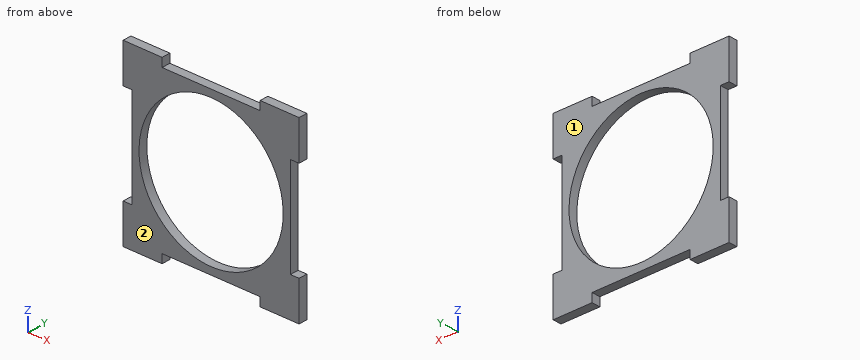
from build123d import *

# Parameters (mm, degrees)
CROQUIS1_R              = 25
SALIENTE_EXTRUIR1_DEPTH = 3


with BuildPart() as part:
    # Croquis1 → Saliente-Extruir1 (new body)
    with BuildSketch(Plane(origin=(0, 0, 0), x_dir=(1, 0, 0), z_dir=(0, 1, 0))):
        Polygon((-27.5, 0), (-27.5, 17), (-30.5, 17), (-30.5, 23.75), (-30.5, 30.5), (-23.75, 30.5), (-17, 30.5), (-17, 27.5), (0, 27.5), (17, 27.5), (17, 30.5), (23.75, 30.5), (30.5, 30.5), (30.5, 23.75), (30.5, 17), (27.5, 17), (27.5, 0), (27.5, -17), (30.5, -17), (30.5, -30.5), (23.75, -30.5), (17, -30.5), (17, -27.5), (0, -27.5), (-17, -27.5), (-17, -30.5), (-23.75, -30.5), (-30.5, -30.5), (-30.5, -23.75), (-30.5, -17), (-27.5, -17), align=None)
        with Locations(Location((0, 0, 0), (0, 0, 270))):
            Circle(CROQUIS1_R, mode=Mode.SUBTRACT)
    extrude(amount=SALIENTE_EXTRUIR1_DEPTH)


solid = part.part
Verification items for the finished model (mm, model axes). Face numbers are marked on the shaded views. Give positions to 0.01 mm unless a question says otherwise; leave off trailing zeros. Loops run counter-clockwise (first coordinate to the right, second up) from the corner with the lowest first, then second, coordinate; pieces in that order, holes last.
1) Thickness scan on line 1 along X through (y, z) = (0.6, 0); line 2 along Z through (x, y) = (0.5, 0.9) (3 decimals); line 3 along Z through (x, y) = (14.5, 0.8). Record the ranges inside material, lowest first.
2) Sectioned sample at C-C, the plane x = 23.5. Enter the section's corners in (y, z), then the cut area to 3 significant figures.
3) Depth check by flat-ended pin: pin 1 Ø0.9 at (x, y) = (3, 1) entering from +Z; pin 2 Ø1.5 at (x, z) = (-23, -8.5) entering from -Y. Enter the tip coordinate at first touch or a pass-through.
4) Sectioned sample at B-B, the plane z = 0. Enter the section's corners in (x, y), then the cut area to 3 significant figures.
5) Draft check along Y on the marked faces 1 and 2. Enter one of: pulls with the +Y half, pulls with the -Y half, needs draft (parallel to the pull), parting line crosses it, or undercut.
6) Sectioned sample at A-A, the plane y = 1.4. Enter the section's corners in (x, z).
Answers:
1. line 1: x = -27.5 to -25, 25 to 27.5
1. line 2: z = -27.5 to -24.995, 24.995 to 27.5
1. line 3: z = -27.5 to -20.37, 20.37 to 27.5
2. outline: (0, -30.5) - (3, -30.5) - (3, -8.53) - (0, -8.53) - close; (0, 8.53) - (3, 8.53) - (3, 30.5) - (0, 30.5) - close
2. area: 132 mm2
3. pin 1: stops at z = 27.5
3. pin 2: stops at y = 0
4. outline: (-27.5, 0) - (-25, 0) - (-25, 3) - (-27.5, 3) - close; (25, 0) - (27.5, 0) - (27.5, 3) - (25, 3) - close
4. area: 15.0 mm2
5. face 1: pulls with the +Y half
5. face 2: pulls with the -Y half
6. outline: (-30.5, -30.5) - (-17, -30.5) - (-17, -27.5) - (17, -27.5) - (17, -30.5) - (30.5, -30.5) - (30.5, -17) - (27.5, -17) - (27.5, 17) - (30.5, 17) - (30.5, 30.5) - (17, 30.5) - (17, 27.5) - (-17, 27.5) - (-17, 30.5) - (-30.5, 30.5) - (-30.5, 17) - (-27.5, 17) - (-27.5, -17) - (-30.5, -17) - close; hole circle Ø50 at (0, 0)
